For this review, use the dimensioned drawing (mm, ordinates from the lowest corner) and the shaded views. Coordinates: 2 decimals unless noted, no trailing zeros. Write each loop counter-clockwise with the first axis right and the second up, starting at its lowest first coordinate (ties: lowest second). Pieces come first, ordered by that corner, then holes. Notation, with made-up numbers: (23, 33) - (39, 33) arc R12 ccw to (39, 47) - close; hole circle Ø8 at (32.25, -29). An arc over 180 degrees is marked (long way). Use one line per item in the form item = value. Start each with the question number.
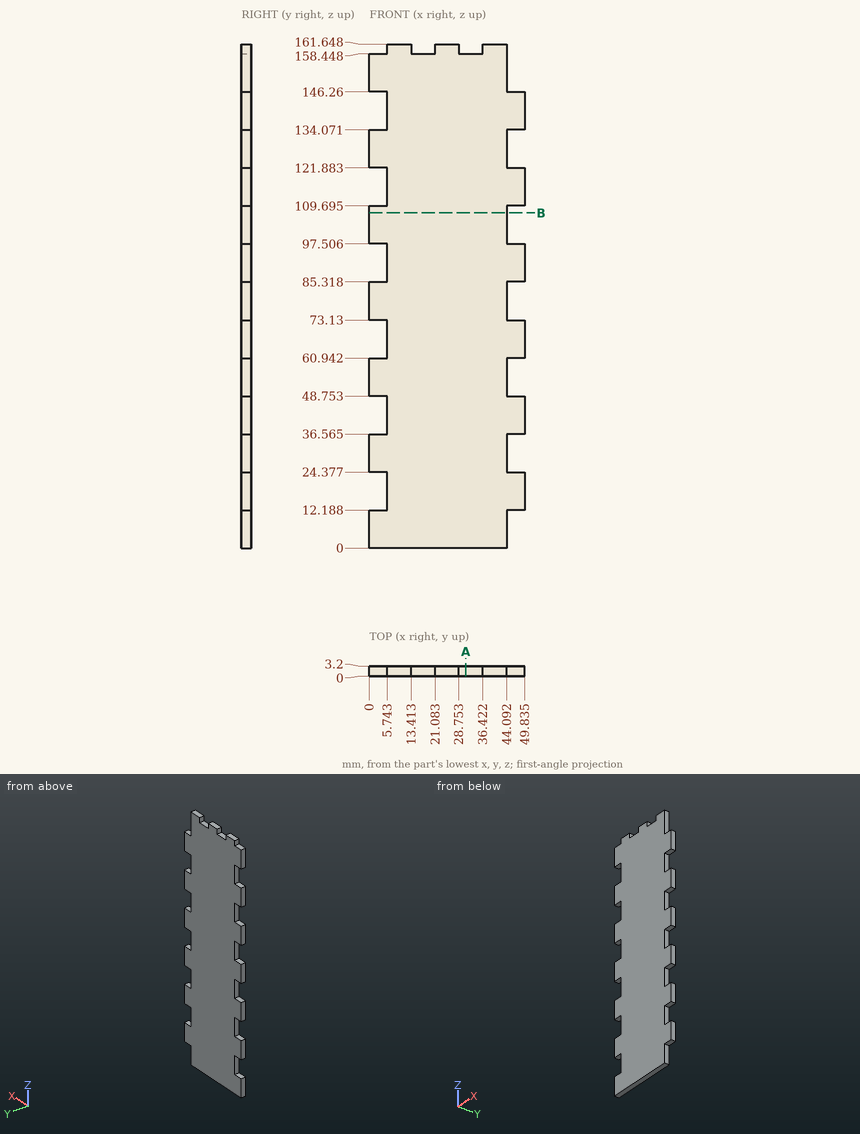
1. Take a section at B-B (z = 107.5). State the section outline as (x, y) points.
2. For P1, Ø1.6, axis at x = 4, y = 1.5, coming from the +Z side; P2, Ø1.6, axis at x = 47.5, y = 2.5, coming from the -Z side; P3, Ø1, axis at y = 1.5, z = 159.5, coming from the +X side, all flat-tipped, find the tip position at first contact; note any pin that passes through.
3. For L1, parallel to Z at x = 18.5, y = 2.45; L2, parallel to X at y = 2.5, z = 86 (1 decimal); L3, parallel to X at y = 0.3, z = 124, list the stretches that pass through material, from the lowest coordinate up.
4. Take a section at A-A (x = 31). State the section outline as (y, z) points.
Returned:
q1.outline = (0, 0) - (44.09, 0) - (44.09, 3.2) - (0, 3.2) - close
q2.P1 = 158.45
q2.P2 = 12.19
q2.P3 = 44.09
q3.L1 = 0 to 158.45
q3.L2 = 5.7 to 49.8
q3.L3 = 0 to 44.09
q4.outline = (0, 0) - (3.2, 0) - (3.2, 158.45) - (0, 158.45) - close
